```python
from build123d import *

# Parameters (mm, degrees)
BOSS_EXTRUDE1_DEPTH = 0.508
SKETCH3_R           = 1.905
CUT_EXTRUDE1_DEPTH  = 1.5080001


with BuildPart() as part:
    # Sketch1 → Boss-Extrude1 (new body)
    with BuildSketch(Plane.XY):
        with BuildLine():
            Line((0, 0), (15.252199682, 0))
            add(Edge.make_bspline(
                [(15.252199682, 0), (15.120704697, 0.830694341), (14.937497846, 1.646944845), (14.553106346, 2.840713056), (14.406511336, 3.233478401), (14.065397829, 4.0056234), (13.872436019, 4.381220548), (13.432237437, 5.09798559), (13.181982939, 5.443027105), (12.622569242, 6.068152419), (12.313627231, 6.349687516), (11.791041042, 6.709189105), (11.607426909, 6.817668629), (11.230562195, 7.003786767), (11.035975482, 7.082401547), (10.633831708, 7.209189667), (10.425174386, 7.257312019), (10.006679556, 7.320082622), (9.795580815, 7.335304029), (9.582738696, 7.335304029)],
                knots=[0, 0, 0, 0, 0.25, 0.25, 0.375, 0.375, 0.5, 0.5, 0.625, 0.625, 0.75, 0.75, 0.8125, 0.8125, 0.875, 0.875, 0.9375, 0.9375, 1, 1, 1, 1], degree=3))
            Line((9.582738696, 7.335304029), (5.669460986, 7.335304029))
            add(Edge.make_bspline(
                [(5.669460986, 7.335304029), (5.243996086, 7.335304029), (4.828702614, 7.274669933), (4.222365546, 7.084743854), (4.024617237, 7.005080674), (3.647485659, 6.819183421), (3.466491387, 6.712483598), (3.118434336, 6.473781927), (2.950963248, 6.341174992), (2.637156438, 6.060474457), (2.489557897, 5.911629159), (2.070541236, 5.44338386), (1.820997709, 5.099528272), (1.159883637, 4.023480986), (0.833207908, 3.254615604), (0.445697358, 2.055038054), (0.334748926, 1.647706186), (0.144996604, 0.828712342), (0.06582017, 0.415806296), (0, 0)],
                knots=[0, 0, 0, 0, 0.125, 0.125, 0.1875, 0.1875, 0.25, 0.25, 0.3125, 0.3125, 0.375, 0.375, 0.5, 0.5, 0.75, 0.75, 0.875, 0.875, 1, 1, 1, 1], degree=3))
        make_face()
    extrude(amount=BOSS_EXTRUDE1_DEPTH)

    # Sketch3 → Cut-Extrude1 (cut, through all)
    with BuildSketch(Plane.XY.offset(0.508)):
        with Locations((7.626099841, 3.667652015)):
            Circle(SKETCH3_R)
    extrude(amount=-CUT_EXTRUDE1_DEPTH, mode=Mode.SUBTRACT)


solid = part.part
```
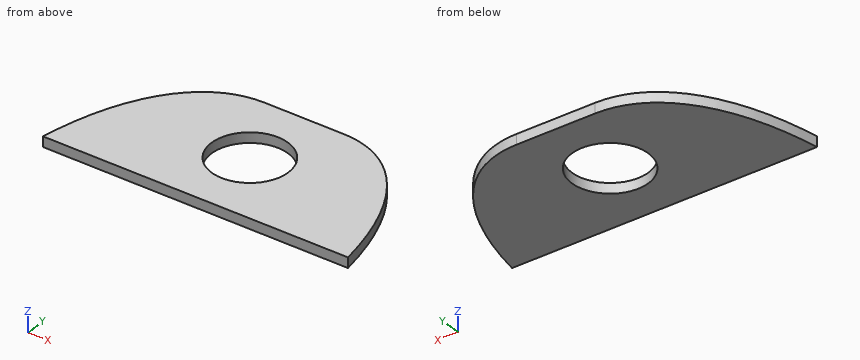
Work out the finished part from the listing and answer in its coordinate system (mm). Coordinates: 2 decimals unless noted, no trailing zeros. Order: outer loops, then holes, each group sorted by start corner. A loop starts at its lowest first (then second) coordinate and runs counter-clockwise, first axis right, second up. Notation, with made-up numbers: M 27,39 L 36,39 A32 cw 36,71 Z; hole C 64.5,-34 d1. An arc over 180 degrees is marked long. Use CSV: the item, a comma, the result in double quotes.
1) Section A-A on x = 9 is taken. Write down the section's boundary in (y, z).
Worked out:
outline,"M 0,0 L 2.35,0 L 2.35,0.51 L 0,0.51 Z; M 4.99,0 L 7.34,0 L 7.34,0.51 L 4.99,0.51 Z"
2) Consider line 1 (Y direction, x = 9.75, z = 0.1); line 2 (X direction, y = 2.25, z = 0.2); line 3 (X direction, y = 2.5, z = 0.45). Determine where each line is inside the solid, lowest interval first. Write a range as [from, to].
Worked out:
line 1,"y = [0, 7.33]"
line 2,"x = [0.51, 6.35], [8.9, 14.74]"
line 3,"x = [0.59, 6.12], [9.13, 14.66]"
3) Section B-B on x = 6.75 is taken. Write down the section's boundary in (y, z).
Worked out:
outline,"M 0,0 L 1.98,0 L 1.98,0.51 L 0,0.51 Z; M 5.36,0 L 7.34,0 L 7.34,0.51 L 5.36,0.51 Z"
